Geometry check sheet. Reference: the model listing, model coordinates, mm. Face numbers are marked on the shaded views. Give positions to 0.01 mm unless a question says otherwise; leave off trailing zeros. Loops run counter-clockwise (first coordinate to the right, second up) from the corner with the lowest first, then second, coordinate; pieces in that order, holes last. Notation, with made-up numbers: (-18, 78) -> (-3, 78) arc R25 ccw to (-3, 92) -> close; hole circle Ø2 at (37, 64). An arc over 180 degrees is marked (long way). One line per item, written item: value. Start each with the question number.
(1) Sectioned sample at C-C, the plane y = 34. Record the cut outline in (x, z).
(2) Scan lines: line 1 along X through (y, z) = (31, 3.4); line 2 along X through (y, z) = (83, 2.7); line 3 along Y through (x, z) = (17.3, 2.15). Record each from-to range of solid material in increasing order. Write a range as from..to.
(3) Sectioned sample at B-B, the plane x = 65. Record the cut outline in (y, z), then the cut area to 3 significant figures.
(4) Sectioned sample at A-A, the plane y = 58.5. Record the cut outline in (x, z).
(5) Draft check along X on the marked faces 1 and 2. Enter one of: pulls with the +X half, pulls with the -X half, needs draft (parallel to the pull), parting line crosses it, or undercut.
(6) Gauge pin test, flat ends, axial feed: pin 1 Ø10 at (x, y) = (34, 101.5) entering from -Z; pin 2 Ø0.6 at (x, z) = (23, 2.5) entering from -Y; pin 3 Ø3 at (y, z) = (38.5, 4.5) entering from -X; pin 4 Ø1.6 at (y, z) = (46.5, 3) entering from +X. Record the tip position at first contact, or that the pin passes through.
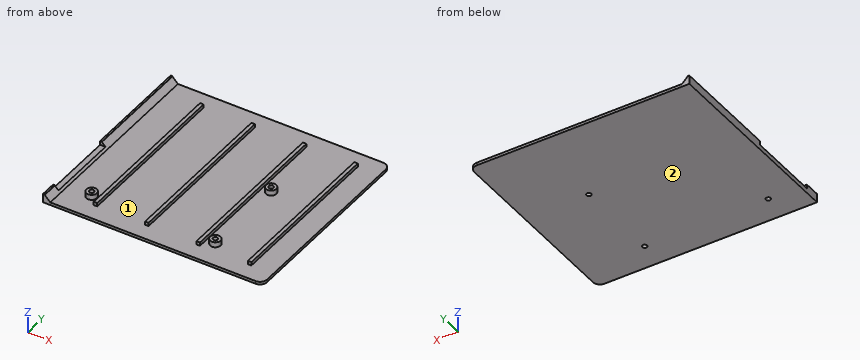
from build123d import *

# Parameters (mm, degrees)
SKETCH_R      = 1.35
PAD_DEPTH     = 1.6
SKETCH001_R   = 3
SKETCH001_R_2 = 1.35
PAD001_DEPTH  = 3
SKETCH002_W   = 2
SKETCH002_H   = 95
PAD002_DEPTH  = 2
SKETCH003_W   = 114
SKETCH003_H   = 5
PAD003_DEPTH  = 1
CHAMFER_SIZE  = 3.19
SKETCH004_W   = 42
SKETCH004_H   = 2.3
POCKET_DEPTH  = 5


with BuildPart() as part:
    # Sketch → Pad (new body)
    with BuildSketch(Plane.XY):
        with BuildLine():
            Line((0, 0), (121, 0))
            ThreePointArc((121, 0), (123.828427, 1.171573), (125, 4))
            Line((125, 4), (125, 110))
            ThreePointArc((125, 110), (123.828427, 112.828427), (121, 114))
            Line((121, 114), (0, 114))
            Line((0, 114), (0, 0))
        make_face()
        with Locations((17.3, 15)):
            Circle(SKETCH_R, mode=Mode.SUBTRACT)
        with Locations((88.3, 64.8)):
            Circle(SKETCH_R, mode=Mode.SUBTRACT)
        with Locations((88.3, 15)):
            Circle(SKETCH_R, mode=Mode.SUBTRACT)
    extrude(amount=PAD_DEPTH)

    # Sketch001 (on Face11 of Pad) → Pad001 (join)
    with BuildSketch(Plane.XY.offset(1.6)):
        with Locations((88.3, 15)):
            Circle(SKETCH001_R)
        with Locations((88.3, 15)):
            Circle(SKETCH001_R_2, mode=Mode.SUBTRACT)
        with Locations((88.3, 64.8)):
            Circle(SKETCH001_R)
        with Locations((88.3, 64.8)):
            Circle(SKETCH001_R_2, mode=Mode.SUBTRACT)
        with Locations((17.3, 15)):
            Circle(SKETCH001_R)
        with Locations((17.3, 15)):
            Circle(SKETCH001_R_2, mode=Mode.SUBTRACT)
    extrude(amount=PAD001_DEPTH)

    # Sketch002 (on Face5 of Pad001) → Pad002 (join)
    with BuildSketch(Plane.XY.offset(1.6)):
        with Locations((23, 57)):
            Rectangle(SKETCH002_W, SKETCH002_H)
        with Locations((52.5, 57)):
            Rectangle(SKETCH002_W, SKETCH002_H)
        with Locations((82, 57)):
            Rectangle(SKETCH002_W, SKETCH002_H)
        with Locations((111.5, 57)):
            Rectangle(SKETCH002_W, SKETCH002_H)
    extrude(amount=PAD002_DEPTH)

    # Sketch003 (on Face2 of Pad002) → Pad003 (join)
    with BuildSketch(Plane(origin=(0, 0, 0), x_dir=(0, -1, 0), z_dir=(-1, 0, 0))):
        with Locations((-57, 2.5)):
            Rectangle(SKETCH003_W, SKETCH003_H)
    extrude(amount=PAD003_DEPTH)

    # Chamfer
    chamfer_edges = [part.edges().sort_by_distance(p)[0] for p in [
        (0, 57, 1.6),
    ]]
    chamfer(chamfer_edges, length=CHAMFER_SIZE)

    # Sketch004 (on Face31 of Chamfer) → Pocket (cut)
    with BuildSketch(Plane(origin=(-1, 0, 0), x_dir=(0, -1, 0), z_dir=(-1, 0, 0))):
        with Locations((-30, 3.85)):
            Rectangle(SKETCH004_W, SKETCH004_H)
    extrude(amount=-POCKET_DEPTH, mode=Mode.SUBTRACT)


solid = part.part
Calculated:
1. outline: (-1, 0) -> (125, 0) -> (125, 1.6) -> (112.5, 1.6) -> (112.5, 3.6) -> (110.5, 3.6) -> (110.5, 1.6) -> (83, 1.6) -> (83, 3.6) -> (81, 3.6) -> (81, 1.6) -> (53.5, 1.6) -> (53.5, 3.6) -> (51.5, 3.6) -> (51.5, 1.6) -> (24, 1.6) -> (24, 3.6) -> (22, 3.6) -> (22, 1.6) -> (3.19, 1.6) -> (2.09, 2.7) -> (-1, 2.7) -> close
2. line 1: x = 22..24, 51.5..53.5, 81..83, 110.5..112.5
2. line 2: x = -1..2.09, 22..24, 51.5..53.5, 81..83, 110.5..112.5
2. line 3: y = 12..13.65, 16.35..18
3. outline: (0, 0) -> (114, 0) -> (114, 1.6) -> (0, 1.6) -> close
3. area: 182 mm2
4. outline: (-1, 0) -> (125, 0) -> (125, 1.6) -> (112.5, 1.6) -> (112.5, 3.6) -> (110.5, 3.6) -> (110.5, 1.6) -> (83, 1.6) -> (83, 3.6) -> (81, 3.6) -> (81, 1.6) -> (53.5, 1.6) -> (53.5, 3.6) -> (51.5, 3.6) -> (51.5, 1.6) -> (24, 1.6) -> (24, 3.6) -> (22, 3.6) -> (22, 1.6) -> (3.19, 1.6) -> (0, 4.79) -> (0, 5) -> (-1, 5) -> close
5. face 1: undercut
5. face 2: needs draft
6. pin 1: stops at z = 0
6. pin 2: stops at y = 9.5
6. pin 3: stops at x = 22
6. pin 4: stops at x = 112.5
